Verification items for the finished model (mm, model axes). A direction names the side the tool comes from. Coordinates: 2 decimals unless noted, no trailing zeros. Order: outer loops, then holes, each group sorted by start corner. A loop starts at its lowest first (then second) coordinate and runs counter-clockwise, first axis right, second up. Notation, with made-up numbers: (17.25, -3.5) -> (46.25, -3.5) arc R23 cw to (46.25, 15.5) -> close; hole circle Ø5 at (6.5, 15). An arc over 180 degrees is marked (long way). Use CSV: the item, a comma, the result in double quotes. Start each with the question number.
1) Sectioned sample at B-B on z = -18. Record the boundary of the cut face in (x, y).
2) Sectioned sample at C-C on y = 37. Record the boundary of the cut face in (x, z).
3) Tool access check on faces 1 (the flat face through (558.107, 301, 337)), 2 (the flat face through (61, 6.35, 321)), 3 (the flat face through (223, 76.2, -50)). Record the directions out of +Z, -Z, +X, -X, +Y, -Y that give a thin tool (end or side, any length) a straight path to the whole face; none if there is none.
4) Release check for a two-part mould opening along X. For faces 4 (the flat face through (-102.293, 301, 349)), 5 (the flat face through (233, 301, 787.4)), 6 (the flat face through (392, 6.35, 321)) record: released by +X, released by -X, zero draft, split by the parting line, or undercut.
5) Sectioned sample at A-A on x = 451.5. Record the boundary of the cut face in (y, z).
6) Scan lines: line 1 along Y through (x, z) = (399, -42.5); line 2 along Y through (x, z) = (331.5, 440.5); line 3 along Z through (x, y) = (181, 46). Record each from-to range of solid material in increasing order.
7) Go/stop test with flat-tipped pins: pin 1 (6 mm diameter, centred on x = 434.5, z = 324, fed in from -Y); pin 2 (1.9 mm diameter, centred on x = 131, y = 3.5, fed in from -Z). Record where each tip stops, or that it passes through.
from build123d import *

# Parameters (mm, degrees)
F0_W     = 3.175
F0_H     = 635
F0_W_2   = 327.025
F0_W_3   = 203.2
F0_H_2   = 508
F0_W_4   = 330.2
F0_H_3   = 147.32
F1_DEPTH = 609.6
F2_DEPTH = 6.35
F3_DEPTH = 76.2


with BuildPart() as f1:
    # F0 (on Front) → F1 (new body)
    with BuildSketch(Plane.XZ):
        Polygon((227.9072425127, -101.6), (227.9072425127, 0), (224.7322425127, 0), (-102.2927574873, 0), (-102.2927574873, -101.6), align=None)
        with Locations((226.3197425127, 317.5)):
            Rectangle(F0_W, F0_H)
        Polygon((231.0822425127, 0), (227.9072425127, 0), (227.9072425127, -101.6), (558.1072425127, -101.6), (558.1072425127, 0), align=None)
        with Locations((229.4947425127, 317.5)):
            Rectangle(F0_W, F0_H)
        with Locations((61.2197425127, 317.5)):
            Rectangle(F0_W_2, F0_H)
        with Locations((62.8072425127, 317.5)):
            Rectangle(F0_W_3, F0_H_2, mode=Mode.SUBTRACT)
        Polygon((224.7322425127, 635), (227.9072425127, 635), (227.9072425127, 640.08), (-102.2927574873, 640.08), (-102.2927574873, 635), align=None)
        Polygon((227.9072425127, 640.08), (227.9072425127, 635), (231.0822425127, 635), (558.1072425127, 635), (558.1072425127, 640.08), align=None)
        with Locations((394.5947425127, 317.5)):
            Rectangle(F0_W_2, F0_H)
        with Locations((393.0072425127, 317.5)):
            Rectangle(F0_W_3, F0_H_2, mode=Mode.SUBTRACT)
        with Locations((62.8072425127, 713.74)):
            Rectangle(F0_W_4, F0_H_3)
        with Locations((393.0072425127, 713.74)):
            Rectangle(F0_W_4, F0_H_3)
        with Locations((62.8072425127, 317.5)):
            Rectangle(F0_W_3, F0_H_2)
        with Locations((393.0072425127, 317.5)):
            Rectangle(F0_W_3, F0_H_2)
    extrude(amount=-F1_DEPTH)

    # F0 (on Front) → F2 (cut)
    with BuildSketch(Plane.XZ):
        with Locations((226.3197425127, 317.5)):
            Rectangle(F0_W, F0_H)
        with Locations((229.4947425127, 317.5)):
            Rectangle(F0_W, F0_H)
        Polygon((224.7322425127, 635), (227.9072425127, 635), (227.9072425127, 640.08), (-102.2927574873, 640.08), (-102.2927574873, 635), align=None)
        Polygon((227.9072425127, 640.08), (227.9072425127, 635), (231.0822425127, 635), (558.1072425127, 635), (558.1072425127, 640.08), align=None)
        with Locations((62.8072425127, 317.5)):
            Rectangle(F0_W_3, F0_H_2)
        with Locations((393.0072425127, 317.5)):
            Rectangle(F0_W_3, F0_H_2)
    extrude(amount=-F2_DEPTH, mode=Mode.SUBTRACT)

    # F0 (on Front) → F3 (cut)
    with BuildSketch(Plane.XZ):
        Polygon((227.9072425127, -101.6), (227.9072425127, 0), (224.7322425127, 0), (-102.2927574873, 0), (-102.2927574873, -101.6), align=None)
        Polygon((231.0822425127, 0), (227.9072425127, 0), (227.9072425127, -101.6), (558.1072425127, -101.6), (558.1072425127, 0), align=None)
    extrude(amount=-F3_DEPTH, mode=Mode.SUBTRACT)


solid = f1.part
Answers follow:
1,outline,"(-102.29, 76.2) -> (558.11, 76.2) -> (558.11, 609.6) -> (-102.29, 609.6) -> close"
2,outline,"(-102.29, 0) -> (558.11, 0) -> (558.11, 787.4) -> (-102.29, 787.4) -> close"
3,face 1,"+Z, -Z, +X, +Y, -Y"
3,face 2,"-Y"
3,face 3,"-Z, +X, -X, -Y"
4,face 4,"released by -X"
4,face 5,"zero draft"
4,face 6,"undercut"
5,outline,"(0, 0) -> (76.2, 0) -> (76.2, -101.6) -> (609.6, -101.6) -> (609.6, 787.4) -> (0, 787.4) -> (0, 640.08) -> (6.35, 640.08) -> (6.35, 635) -> (0, 635) -> (0, 571.5) -> (6.35, 571.5) -> (6.35, 63.5) -> (0, 63.5) -> close"
6,line 1,"y = 76.2 to 609.6"
6,line 2,"y = 6.35 to 609.6"
6,line 3,"z = 0 to 787.4"
7,pin 1,"stops at y = 6.35"
7,pin 2,"stops at z = 0"
